from build123d import *

# Parameters (mm, degrees)
SKETCH1_W               = 10
SKETCH1_H               = 3.1
SKETCH1_R               = 5.75
SKETCH1_R_2             = 7.6
BOSS_EXTRUDE1_DEPTH     = 3
SKETCH2_W               = 5.2
SKETCH2_H               = 2.5
SKETCH2_W_2             = 3.2
SKETCH2_H_2             = 10.5
CUT_EXTRUDE1_DEPTH      = 1
CUT_EXTRUDE1_DEPTH_BACK = 4


with BuildPart() as part:
    # Sketch1 → Boss-Extrude1 (new body)
    with BuildSketch(Plane(origin=(0, 0, 0), x_dir=(0, 0, -1), z_dir=(1, 0, 0))):
        Polygon((0, 43), (0, 0), (12.5, 0), (12.5, -9), (27.5, -9), (27.5, 0), (68.19375928, 0), (68.19375928, 43), (45.462506187, 43), (45.462506187, 46), (22.731253093, 46), (22.731253093, 43), align=None)
        with Locations((20, -4.65)):
            Rectangle(SKETCH1_W, SKETCH1_H, mode=Mode.SUBTRACT)
        with Locations((17.5, 14.8978)):
            Circle(SKETCH1_R, mode=Mode.SUBTRACT)
        with Locations((50.69375928, 21)):
            Circle(SKETCH1_R_2, mode=Mode.SUBTRACT)
    extrude(amount=BOSS_EXTRUDE1_DEPTH)

    # Sketch2 → Cut-Extrude1 (cut, two sides)
    with BuildSketch(Plane(origin=(3, 0, 0), x_dir=(0, 0, -1), z_dir=(1, 0, 0))) as cut_extrude1_sk:
        with BuildLine():
            Line((15, 20.075878794), (15, 23.075878794))
            Line((15, 23.075878794), (20, 23.075878794))
            Line((20, 23.075878794), (20, 20.075878794))
            ThreePointArc((20, 20.075878794), (17.5, 20.6478), (15, 20.075878794))
        make_face()
        with Locations((34.09687964, 41.575)):
            Rectangle(SKETCH2_W, SKETCH2_H)
        with Locations((34.09687964, 40.75)):
            Rectangle(SKETCH2_W_2, SKETCH2_H_2)
    extrude(amount=CUT_EXTRUDE1_DEPTH, mode=Mode.SUBTRACT)
    extrude(cut_extrude1_sk.sketch, amount=-CUT_EXTRUDE1_DEPTH_BACK, mode=Mode.SUBTRACT)


solid = part.part
Model file for the job. Use its own axes, mm. A direction names the side the tool comes from. Round coordinates to 2 decimals unless told otherwise and drop trailing zeros. Loops run counter-clockwise (first coordinate to the right, second up) from the corner with the lowest first, then second, coordinate; pieces in that order, holes last.
1. Drop flat-ended pins along their axis: P1, Ø1.5, axis at x = 1, y = 44, coming from the -Z side; P2, Ø10, axis at y = 31.5, z = -25, coming from the -X side; P3, Ø0.9, axis at x = 1.5, z = -58, coming from the +Y side; P4, Ø0.9, axis at x = 1, y = -4.5, coming from the -Z side. Give the stop position or say it passes through.
Check values:
P1: stops at z = -45.46
P2: stops at x = 0
P3: stops at y = 43
P4: stops at z = -27.5
2. Wall check: probe 1 along Y at (x, z) = (1.3, -17.5); probe 2 along Z at (x, y) = (1.85, 14); probe 3 along Z at (x, y) = (2, 38.5). Give the ranges that are in metal, low to high.
Check values:
probe 1: y = -9 to -6.2, -3.1 to 9.15, 23.08 to 43
probe 2: z = -68.19 to -53.65, -47.73 to -23.18, -11.82 to 0
probe 3: z = -68.19 to -35.7, -32.5 to 0
3. Mould opens along Z. For faces 6 (the flat face through (1, -9, -20)), 7 (the flat face through (2, 22, -15)), 8 (the flat face through (1, 21, -68.194)) say: +Z half, -Z half, draft (parallel to the pull), parting line (faces both ways), or undercut.
Check values:
face 6: draft
face 7: undercut
face 8: -Z half
4. Band-saw the part on C-C, the plane x = 2.5. Count the separate pieces of the cut face and the enclosed holes in it, and give its area (3 significant figures).
Check values:
separate pieces: 1
enclosed holes: 3
area: 2,770 mm2
5. Band-saw the part on D-D, the plane z = -17.5. List the corners of the cut face in (x, y).
Check values:
outline: (0, -9) - (3, -9) - (3, -6.2) - (0, -6.2) - close; (0, -3.1) - (3, -3.1) - (3, 9.15) - (0, 9.15) - close; (0, 23.08) - (3, 23.08) - (3, 43) - (0, 43) - close
6. Tool access for faces 1 (the flat face through (1, 44, -45.463)), 2 (the flat face through (1, -3.1, -20)), 3 (the flat face through (2, 44, -35.697)), 4 (the flat face through (1, -5, -27.5)), 5 (the flat face through (1, 45, -22.731)): list every direction of +Z, -Z, +X, -X, +Y, -Y with a clear straight run to the whole face (end or side of a thin tool).
Check values:
face 1: -Z, +X, -X, +Y
face 2: +X, -X
face 3: +X, -X, +Y
face 4: -Z, +X, -X, -Y
face 5: +Z, +X, -X, +Y
7. Band-saw the part on A-A, the plane y = 21. List the corners of the cut face in (x, z), and give its area (3 significant figures).
Check values:
outline: (0, -68.19) - (3, -68.19) - (3, -58.29) - (0, -58.29) - close; (0, -43.09) - (3, -43.09) - (3, -20) - (0, -20) - close; (0, -15) - (3, -15) - (3, 0) - (0, 0) - close
area: 144 mm2
8. Band-saw the part on B-B, the plane y = 36.5. List the corners of the cut face in (x, z), and give its area (3 significant figures).
Check values:
outline: (0, -68.19) - (3, -68.19) - (3, -35.7) - (0, -35.7) - close; (0, -32.5) - (3, -32.5) - (3, 0) - (0, 0) - close
area: 195 mm2
